Here's how the part is built. I have some questions about the finished solid (model axes, mm). Coordinates: 2 decimals unless noted, no trailing zeros. Order: outer loops, then holes, each group sorted by start corner. A loop starts at its lowest first (then second) coordinate and runs counter-clockwise, first axis right, second up. Notation, with made-up numbers: (21.25, 14.5) -> (73.25, 14.5) arc R21 ccw to (73.25, 20.5) -> close; hole circle Ø6 at (68, -32). An arc over 180 degrees is marked (long way). One line per item, written item: value. Start each with the question number.
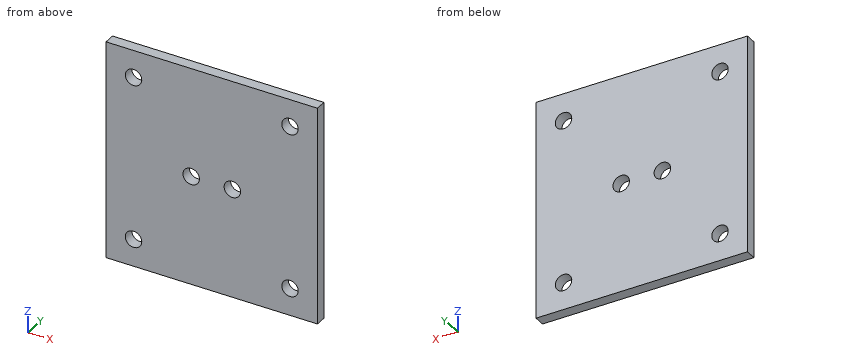
```python
from build123d import *

# Parameters (mm, degrees)
SKETCH1_W           = 77
SKETCH1_H           = 80
SKETCH1_R           = 3
BOSS_EXTRUDE1_DEPTH = 2


with BuildPart() as part:
    # Sketch1 → Boss-Extrude1 (new, symmetric)
    with BuildSketch(Plane(origin=(0, 0, 0), x_dir=(1, 0, 0), z_dir=(0, 1, 0))):
        Rectangle(SKETCH1_W, SKETCH1_H)
        with Locations(Location((-7.5, 0, 0), (0, 0, 270))):
            Circle(SKETCH1_R, mode=Mode.SUBTRACT)
        with Locations(Location((7.5, 0, 0), (0, 0, 270))):
            Circle(SKETCH1_R, mode=Mode.SUBTRACT)
        with Locations(Location((-28.5, 30, 0), (0, 0, 270))):
            Circle(SKETCH1_R, mode=Mode.SUBTRACT)
        with Locations(Location((28.5, 30, 0), (0, 0, 270))):
            Circle(SKETCH1_R, mode=Mode.SUBTRACT)
        with Locations(Location((28.5, -30, 0), (0, 0, 90))):
            Circle(SKETCH1_R, mode=Mode.SUBTRACT)
        with Locations(Location((-28.5, -30, 0), (0, 0, 90))):
            Circle(SKETCH1_R, mode=Mode.SUBTRACT)
    extrude(amount=BOSS_EXTRUDE1_DEPTH, both=True)


solid = part.part
```
Q1. Imagine slicing it at D-D (x = -28.5). Write out the boundary of the cut face in (y, z), plus the area to 3 significant figures.
Q2. Imagine slicing it at A-A (x = -7.5). Write out the boundary of the cut face in (y, z), plus the area to 3 significant figures.
Q3. I need wall thicknesses on line 1 (X direction, y = -0.2, z = 30); line 2 (Z direction, x = -30.5, y = -0.65); line 3 (X direction, y = -1.2, z = 32). Which ranges of each line are inside material? Lowest first, please.
Q4. Imagine slicing it at B-B (z = 30). Write out the boundary of the cut face in (x, y).
Q5. For P1, Ø5, axis at x = 7.5, z = 0, coming from the +Y side, with a flat end and sliding along its axis, tell me the tip position at first contact or that it passes through.
Q6. Imagine slicing it at C-C (y = -0.75). Write out the boundary of the cut face in (x, z), plus the area to 3 significant figures.
Completed:
1. outline: (-2, -40) -> (2, -40) -> (2, -33) -> (-2, -33) -> close; (-2, -27) -> (2, -27) -> (2, 27) -> (-2, 27) -> close; (-2, 33) -> (2, 33) -> (2, 40) -> (-2, 40) -> close
1. area: 272 mm2
2. outline: (-2, -40) -> (2, -40) -> (2, -3) -> (-2, -3) -> close; (-2, 3) -> (2, 3) -> (2, 40) -> (-2, 40) -> close
2. area: 296 mm2
3. line 1: x = -38.5 to -31.5, -25.5 to 25.5, 31.5 to 38.5
3. line 2: z = -40 to -32.24, -27.76 to 27.76, 32.24 to 40
3. line 3: x = -38.5 to -30.74, -26.26 to 26.26, 30.74 to 38.5
4. outline: (-38.5, -2) -> (-31.5, -2) -> (-31.5, 2) -> (-38.5, 2) -> close; (-25.5, -2) -> (25.5, -2) -> (25.5, 2) -> (-25.5, 2) -> close; (31.5, -2) -> (38.5, -2) -> (38.5, 2) -> (31.5, 2) -> close
5. P1: passes through
6. outline: (-38.5, -40) -> (38.5, -40) -> (38.5, 40) -> (-38.5, 40) -> close; hole circle Ø6 at (-28.5, -30); hole circle Ø6 at (-28.5, 30); hole circle Ø6 at (-7.5, 0); hole circle Ø6 at (7.5, 0); hole circle Ø6 at (28.5, -30); hole circle Ø6 at (28.5, 30)
6. area: 5,990 mm2
